Verification items for the finished model (mm, model axes). A direction names the side the tool comes from. Round coordinates to 2 decimals unless told otherwise and drop trailing zeros. Order: outer loops, then holes, each group sorted by start corner. A loop starts at its lowest first (then second) coordinate and runs counter-clockwise, first axis right, second up. Notation, with made-up numbers: M -13.5,43 L 11.5,43 A23 cw 11.5,51 Z; hole C -21.5,-2 d1. An arc over 180 degrees is marked long. Use one line per item in the form item = value. Start each with the question number.
Item 1: Tool access check on faces 1 (the flat face through (-2, 3, 4)), 2 (the cylindrical face through (73.99, 1.52, 12.85)). Record the directions out of +Z, -Z, +X, -X, +Y, -Y that give a thin tool (end or side, any length) a straight path to the whole face; none if there is none.
Item 2: Cross-section at D-D on x = -5.5. Enter the section's corners in (y, z), then the cut area to 3 significant figures.
Item 3: Cross-section at A-A on z = 14. Enter the section's corners in (x, y), then the cut area to 3 significant figures.
Item 4: Release check for a two-part mould opening along Z. For faces 3 (the cylindrical face through (103.58, 1.48, 72.65)), 4 (the cylindrical face through (-90.42, 1.48, 72.65)), 5 (the flat face through (-2, 0, 4)), 6 (the cylindrical face through (-73.99, 1.52, 12.85)) record: +Z half, -Z half, draft (parallel to the pull), parting line (faces both ways), or undercut.
Item 5: Thickness scan on probe 1 along X at (y, z) = (2.3, 60); probe 2 along X at (y, z) = (1.65, 59); probe 3 along Z at (x, y) = (0, 1.4). Record the ranges inside material, lowest first. Write a range as [from, to].
Item 6: Cross-section at C-C on y = 2.55. Count the separate pieces of the cut face and the enclosed holes in it, then the cut area to 3 significant figures.
Item 7: Cross-section at B-B on x = 97. Enter the section's corners in (y, z).
from build123d import *

# Parameters (mm, degrees)
SKETCH1_R           = 1.65
SKETCH1_R_2         = 14.26
BOSS_EXTRUDE1_DEPTH = 3
FILLET1_R           = 10


with BuildPart() as part:
    # Sketch1 → Boss-Extrude1 (new body)
    with BuildSketch(Plane(origin=(0, 0, 0), x_dir=(1, 0, 0), z_dir=(0, 1, 0))):
        with BuildLine():
            Line((-77, -10), (77, -10))
            Line((77, -10), (77, -60))
            ThreePointArc((77, -60), (97, -80), (117, -60))
            Line((117, -60), (117, 10))
            Line((117, 10), (-117, 10))
            Line((-117, 10), (-117, -60))
            ThreePointArc((-117, -60), (-97, -80), (-77, -60))
            Line((-77, -60), (-77, -10))
        make_face()
        with Locations((76.2, 0)):
            Circle(SKETCH1_R, mode=Mode.SUBTRACT)
        with Locations((-76.2, 0)):
            Circle(SKETCH1_R, mode=Mode.SUBTRACT)
        with Locations((-50.8, 0)):
            Circle(SKETCH1_R, mode=Mode.SUBTRACT)
        with Locations((-25.4, 0)):
            Circle(SKETCH1_R, mode=Mode.SUBTRACT)
        Circle(SKETCH1_R, mode=Mode.SUBTRACT)
        with Locations((25.4, 0)):
            Circle(SKETCH1_R, mode=Mode.SUBTRACT)
        with Locations((50.8, 0)):
            Circle(SKETCH1_R, mode=Mode.SUBTRACT)
        with Locations((-101.6, 0)):
            Circle(SKETCH1_R, mode=Mode.SUBTRACT)
        with Locations((101.6, 0)):
            Circle(SKETCH1_R, mode=Mode.SUBTRACT)
        with Locations((-97, -60)):
            Circle(SKETCH1_R_2, mode=Mode.SUBTRACT)
        with Locations((97, -60)):
            Circle(SKETCH1_R_2, mode=Mode.SUBTRACT)
    extrude(amount=BOSS_EXTRUDE1_DEPTH)

    # Fillet1
    fillet1_edges = [part.edges().sort_by_distance(p)[0] for p in [
        (-77, 1.5, 10),
        (-117, 1.5, -10),
        (117, 1.5, -10),
        (77, 1.5, 10),
    ]]
    fillet(fillet1_edges, radius=FILLET1_R)


solid = part.part
Output values:
q1.face_1 = +Z, -Z, +X, -X, +Y
q1.face_2 = +Z, +Y, -Y
q2.outline = M 0,-10 L 3,-10 L 3,10 L 0,10 Z
q2.area = 60.0 mm2
q3.outline = M -117,0 L -75,0 L -75,3 L -117,3 Z; M 75,0 L 117,0 L 117,3 L 75,3 Z
q3.area = 252 mm2
q4.face_3 = undercut
q4.face_4 = undercut
q4.face_5 = draft
q4.face_6 = +Z half
q5.probe_1 = [-117, -111.26], [-82.74, -77], [77, 82.74], [111.26, 117]
q5.probe_2 = [-117, -111.22], [-82.78, -77], [77, 82.78], [111.22, 117]
q5.probe_3 = [-10, -1.65], [1.65, 10]
q6.separate_pieces = 1
q6.enclosed_holes = 11
q6.area = 8,580 mm2
q7.outline = M 0,-10 L 3,-10 L 3,45.74 L 0,45.74 Z; M 0,74.26 L 3,74.26 L 3,80 L 0,80 Z
